Build history of the part. All positions in model axes, mm. Face numbers are marked on the shaded views. Give positions to 0.01 mm unless a question says otherwise; leave off trailing zeros. Loops run counter-clockwise (first coordinate to the right, second up) from the corner with the lowest first, then second, coordinate; pieces in that order, holes last. Notation, with made-up numbers: (37.5, 50) -> (41.5, 50) arc R37 cw to (41.5, 86) -> close; hole circle Ø8 at (29, -29.5). An arc over 180 degrees is marked (long way). One line per question, with ' | ' between items. Start each with the question number.
(1) Slice it at B-B, the plane z = 24. Write the cut outline in (x, y), then the cut area to 3 significant figures.
(2) Flat gauge pins, fed straight in: pin 1 Ø3 at (y, z) = (19, 20.5) entering from -X; pin 2 Ø4 at (x, y) = (11.35, -2.04) entering from -Z; pin 3 Ø2 at (y, z) = (21, 20) entering from +X. Where does each tip first touch, or does it go through?
(3) Slice it at C-C, the plane x = 35. Give the number of separate pieces and of enclosed holes in the cut face, then the cut area to 3 significant figures.
(4) Drill centre lines: L1, parallel to X at y = 28, z = 27.5; L2, parallel to Z at x = 36, y = 11; L3, parallel to Y at x = 32, z = 23. Where is each one in solid material? Low to high. Write a range as from..to.
(5) Mould opens along X. For the marked faces 1, 2 and 3 say: pulls with the +X half, pulls with the -X half, needs draft (parallel to the pull), parting line crosses it, or undercut.
(6) Slice it at A-A, the plane z = 6. Write the cut outline in (x, y), then the cut area to 3 significant figures.
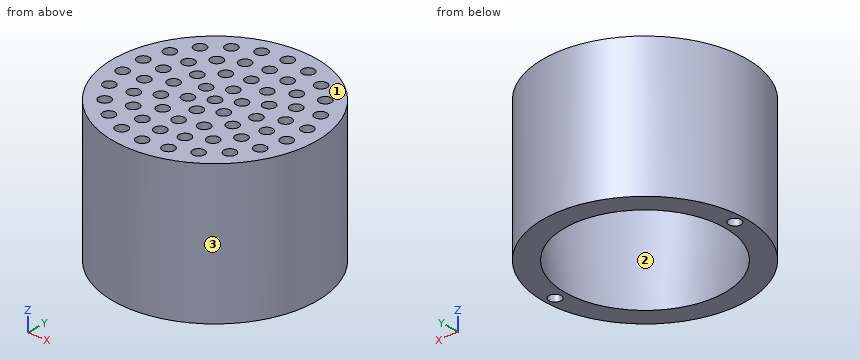
```python
from build123d import *

# Parameters (mm, degrees)
ESQUISSE1_R             = 25.4
BOSS_EXTRU_1_DEPTH      = 25
ESQUISSE6_R             = 1.55
ENL_V_MAT_EXTRU_4_DEPTH = 11
ESQUISSE8_R             = 25.4
BOSS_EXTRU_3_DEPTH      = 10
ESQUISSE9_R             = 1.5
ENL_V_MAT_EXTRU_5_DEPTH = 10


with BuildPart() as part:
    # Esquisse1 → Boss.-Extru.1 (new body)
    with BuildSketch(Plane.XY):
        with Locations((16.625210007, 7.108710486)):
            Circle(ESQUISSE1_R)
    extrude(amount=BOSS_EXTRU_1_DEPTH)

    # Esquisse6 → Enlèv. mat.-Extru.4 (cut)
    with BuildSketch(Plane(origin=(0, 0, 0), x_dir=(-1, 0, 0), z_dir=(0, 0, -1))):
        with Locations((-39.525210007, 7.108710486)):
            Circle(ESQUISSE6_R)
        with Locations((6.274789993, 7.108710486)):
            Circle(ESQUISSE6_R)
    extrude(amount=-ENL_V_MAT_EXTRU_4_DEPTH, mode=Mode.SUBTRACT)

    # Esquisse8 → Boss.-Extru.3 (add)
    with BuildSketch(Plane.XY.offset(25)):
        with Locations((16.625210007, 7.108710486)):
            Circle(ESQUISSE8_R)
    extrude(amount=BOSS_EXTRU_3_DEPTH)

    # Esquisse9 → Enlèv. mat.-Extru.5 (cut)
    with BuildSketch(Plane.XY.offset(35)):
        with Locations((16.625210007, 7.108710486)):
            Circle(ESQUISSE9_R)
        with Locations((16.625210007, 12.388710486)):
            Circle(ESQUISSE9_R)
        with Locations((21.197824139, 9.748710486)):
            Circle(ESQUISSE9_R)
        with Locations((21.197824139, 4.468710486)):
            Circle(ESQUISSE9_R)
        with Locations((16.625210007, 1.828710486)):
            Circle(ESQUISSE9_R)
        with Locations((12.052595875, 4.468710486)):
            Circle(ESQUISSE9_R)
        with Locations((12.052595875, 9.748710486)):
            Circle(ESQUISSE9_R)
        with Locations((16.625210007, 17.668710486)):
            Circle(ESQUISSE9_R)
        with Locations((21.905210007, 16.25393875)):
            Circle(ESQUISSE9_R)
        with Locations((25.770438271, 12.388710486)):
            Circle(ESQUISSE9_R)
        with Locations((27.185210007, 7.108710486)):
            Circle(ESQUISSE9_R)
        with Locations((25.770438271, 1.828710486)):
            Circle(ESQUISSE9_R)
        with Locations((21.905210007, -2.036517778)):
            Circle(ESQUISSE9_R)
        with Locations((16.625210007, -3.451289514)):
            Circle(ESQUISSE9_R)
        with Locations((11.345210007, -2.036517778)):
            Circle(ESQUISSE9_R)
        with Locations((7.479981743, 1.828710486)):
            Circle(ESQUISSE9_R)
        with Locations((6.065210007, 7.108710486)):
            Circle(ESQUISSE9_R)
        with Locations((7.479981743, 12.388710486)):
            Circle(ESQUISSE9_R)
        with Locations((11.345210007, 16.25393875)):
            Circle(ESQUISSE9_R)
        with Locations((16.625210007, 22.948710486)):
            Circle(ESQUISSE9_R)
        with Locations((22.042809078, 21.993441599)):
            Circle(ESQUISSE9_R)
        with Locations((26.806965745, 19.242854465)):
            Circle(ESQUISSE9_R)
        with Locations((30.343052403, 15.028710486)):
            Circle(ESQUISSE9_R)
        with Locations((32.224564815, 9.85929762)):
            Circle(ESQUISSE9_R)
        with Locations((32.224564815, 4.358123352)):
            Circle(ESQUISSE9_R)
        with Locations((30.343052403, -0.811289514)):
            Circle(ESQUISSE9_R)
        with Locations((26.806965745, -5.025433493)):
            Circle(ESQUISSE9_R)
        with Locations((22.042809078, -7.776020627)):
            Circle(ESQUISSE9_R)
        with Locations((16.625210007, -8.731289514)):
            Circle(ESQUISSE9_R)
        with Locations((11.207610937, -7.776020627)):
            Circle(ESQUISSE9_R)
        with Locations((6.44345427, -5.025433493)):
            Circle(ESQUISSE9_R)
        with Locations((2.907367612, -0.811289514)):
            Circle(ESQUISSE9_R)
        with Locations((1.0258552, 4.358123352)):
            Circle(ESQUISSE9_R)
        with Locations((1.0258552, 9.85929762)):
            Circle(ESQUISSE9_R)
        with Locations((2.907367612, 15.028710486)):
            Circle(ESQUISSE9_R)
        with Locations((6.44345427, 19.242854465)):
            Circle(ESQUISSE9_R)
        with Locations((11.207610937, 21.993441599)):
            Circle(ESQUISSE9_R)
        with Locations((16.625210007, 28.228710486)):
            Circle(ESQUISSE9_R)
        with Locations((22.575401608, 27.373202089)):
            Circle(ESQUISSE9_R)
        with Locations((28.043544072, 24.875985099)):
            Circle(ESQUISSE9_R)
        with Locations((32.586641018, 20.939369187)):
            Circle(ESQUISSE9_R)
        with Locations((35.836637749, 15.882275561)):
            Circle(ESQUISSE9_R)
        with Locations((37.53023886, 10.11439987)):
            Circle(ESQUISSE9_R)
        with Locations((37.53023886, 4.103021102)):
            Circle(ESQUISSE9_R)
        with Locations((35.836637749, -1.664854589)):
            Circle(ESQUISSE9_R)
        with Locations((32.586641018, -6.721948215)):
            Circle(ESQUISSE9_R)
        with Locations((28.043544072, -10.658564127)):
            Circle(ESQUISSE9_R)
        with Locations((22.575401608, -13.155781117)):
            Circle(ESQUISSE9_R)
        with Locations((16.625210007, -14.011289514)):
            Circle(ESQUISSE9_R)
        with Locations((10.675018407, -13.155781117)):
            Circle(ESQUISSE9_R)
        with Locations((5.206875943, -10.658564127)):
            Circle(ESQUISSE9_R)
        with Locations((0.663778997, -6.721948215)):
            Circle(ESQUISSE9_R)
        with Locations((-2.586217734, -1.664854589)):
            Circle(ESQUISSE9_R)
        with Locations((-4.279818845, 4.103021102)):
            Circle(ESQUISSE9_R)
        with Locations((-4.279818845, 10.11439987)):
            Circle(ESQUISSE9_R)
        with Locations((-2.586217734, 15.882275561)):
            Circle(ESQUISSE9_R)
        with Locations((0.663778997, 20.939369187)):
            Circle(ESQUISSE9_R)
        with Locations((5.206875943, 24.875985099)):
            Circle(ESQUISSE9_R)
        with Locations((10.675018407, 27.373202089)):
            Circle(ESQUISSE9_R)
    extrude(amount=-ENL_V_MAT_EXTRU_5_DEPTH, mode=Mode.SUBTRACT)

    # Esquisse12 → Enlèvement de matière-Révolution1 (revolve, cut)
    with BuildSketch(Plane(origin=(16.625210007, 0, 0), x_dir=(0, 0, -1), z_dir=(1, 0, 0))):
        Polygon((0, 7.108710486), (0, 27.108710486), (-25, 30.108710486), (-25, 7.108710486), align=None)
    revolve(axis=Axis((16.625210007, 7.108710486, 25), (0, 0, -1)), mode=Mode.SUBTRACT)


solid = part.part
```
Final values:
1) outline: circle Ø50.8 at (16.63, 7.11); hole circle Ø45.76 at (16.63, 7.11) | area: 382 mm2
2) pin 1: x = -6.55 | pin 2: z = 25 | pin 3: x = 38.51
3) separate pieces: 3 | enclosed holes: 0 | area: 624 mm2
4) L1: 2.18..9.31, 12.04..15.14, 18.11..21.21, 23.94..31.07 | L2: 25..35 | L3: -13.11..-9.67, 23.89..27.33
5) face 1: needs draft | face 2: undercut | face 3: parting line crosses it
6) outline: circle Ø50.8 at (16.63, 7.11); hole circle Ø3.1 at (-6.27, 7.11); hole circle Ø41.44 at (16.63, 7.11); hole circle Ø3.1 at (39.53, 7.11) | area: 663 mm2
